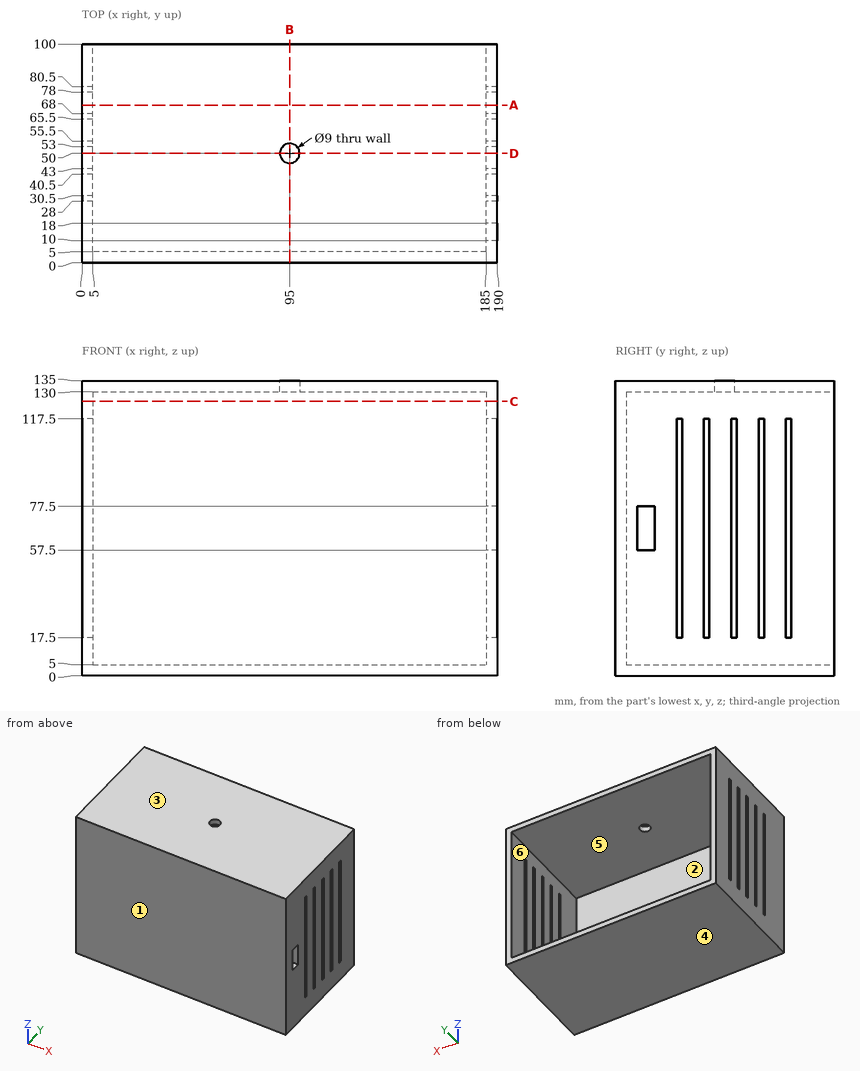
Job drawing, mm, ordinate dimensions from the low corner. One solid piece. A direction names the side the tool comes from. Coordinates: 2 decimals unless noted, no trailing zeros. Write each loop counter-clockwise with the first axis right and the second up, starting at its lowest first coordinate (ties: lowest second). Pieces come first, ordered by that corner, then holes.
Item 1: Slice it at C-C (z = 125.5). Write the cut outline in (x, y), and give its area (3 significant figures).
Item 2: Slice it at A-A (y = 72). Write the cut outline in (x, z).
Item 3: Pin check, flat tip, straight feed: pin 1 (6 mm diameter, centred on x = 120, z = 35, fed in from +Y). Stop position of the tip, or through.
Item 4: Probe line 1 (Z direction, x = 79, y = 42.5); line 2 (X direction, y = 21.5, z = 62.5); line 3 (Y direction, x = 95, z = 131.25). List the from-to ranges inside material, lowest first.
Item 5: Which spindle directions (+Z, -Z, +X, -X, +Y, -Y) get a long thin tool onto all of the face, cutting with end or side? Do the marked faces 1 and 2. Say none if no direction does.
Item 6: Slice it at D-D (y = 50). Write the cut outline in (x, z).
Item 7: Mould opens along Z. For the marked faces 3, 4, 5 and 6 say: released by +Z, released by -Z, zero draft, split by the parting line, or undercut.
Item 8: Slice it at B-B (x = 95). Write the cut outline in (y, z).
Results found:
1. outline: (0, 0) - (190, 0) - (190, 100) - (185, 100) - (185, 5) - (5, 5) - (5, 100) - (0, 100) - close
1. area: 1,900 mm2
2. outline: (0, 0) - (190, 0) - (190, 135) - (0, 135) - close; hole (5, 5) - (185, 5) - (185, 130) - (5, 130) - close
3. pin 1: stops at y = 5
4. line 1: z = 0 to 5, 130 to 135
4. line 2: x = 0 to 5, 185 to 190
4. line 3: y = 0 to 45.5, 54.5 to 100
5. face 1: +Z, -Z, +X, -X, -Y
5. face 2: +Y
6. outline: (0, 0) - (190, 0) - (190, 135) - (99.5, 135) - (99.5, 130) - (185, 130) - (185, 5) - (5, 5) - (5, 130) - (90.5, 130) - (90.5, 135) - (0, 135) - close
7. face 3: released by +Z
7. face 4: released by -Z
7. face 5: undercut
7. face 6: undercut
8. outline: (0, 0) - (100, 0) - (100, 5) - (5, 5) - (5, 130) - (45.5, 130) - (45.5, 135) - (0, 135) - close; (54.5, 130) - (100, 130) - (100, 135) - (54.5, 135) - close
